Input: part model. Units: mm. Frame: model coordinates. Round coordinates to 2 decimals unless told otherwise and drop trailing zeros. Loops run counter-clockwise (first coordinate to the right, second up) from the corner with the lowest first, then second, coordinate; pieces in that order, holes last. Notation, with made-up numbers: (-32, -29) -> (-15, -29) arc R21 ccw to (-15, 2) -> close; hole circle Ø11 at (-27, -30.75). An arc over 180 degrees is marked (long way). Answer in a Markdown table with one row per item. Add a question column.
Q1. Section A-A, the plane x = -123. Output: boundary loops of the cut face in (y, z) (3 decimals).
Q2. Section C-C, the plane x = 107.5. Output: boundary loops of the cut face in (y, z) (3 decimals).
Q3. Ray query, L1, parallel to Z at x = 114.3, y = 9.5; L2, parallel to X at y = 9.75, z = -78. Return the intervals inside material, ascending. Write a range as from..to.
Q4. Section B-B, the plane y = 10.5. Give the number of separate pieces and of enclosed holes in the cut face, and give its area (3 significant figures).
Q5. Mould query, pull axis X, two halves, no side actions, for faces 1 (the face through (103.77, 7.83, -96.84)), 2 (the face through (-152.4, 8, 8)), 3 (the face through (-2, 0, 5)), 4 (the face through (152.4, 8, 8)). Classes: pulls with the +X half, pulls with the -X half, needs draft (parallel to the pull), parting line crosses it, or undercut.
```python
from build123d import *

# Parameters (mm, degrees)
SKETCH1_W           = 304.8
SKETCH1_H           = 266.7
SKETCH1_R           = 14.2875
BOSS_EXTRUDE1_DEPTH = 15.875
SKETCH2_W           = 304.8
SKETCH2_H           = 12.7
CUT_EXTRUDE1_DEPTH  = 16.875


with BuildPart() as part:
    # Sketch1 → Boss-Extrude1 (new body)
    with BuildSketch(Plane(origin=(0, 0, 0), x_dir=(1, 0, 0), z_dir=(0, 1, 0))):
        Rectangle(SKETCH1_W, SKETCH1_H)
        with Locations((-114.3, 87.180661253)):
            Circle(SKETCH1_R, mode=Mode.SUBTRACT)
        with Locations((114.3, 87.180661253)):
            Circle(SKETCH1_R, mode=Mode.SUBTRACT)
    extrude(amount=BOSS_EXTRUDE1_DEPTH)

    # Sketch2 → Cut-Extrude1 (cut, through all)
    with BuildSketch(Plane(origin=(0, 15.875, 0), x_dir=(1, 0, 0), z_dir=(0, 1, 0))):
        with Locations((0, 127)):
            Rectangle(SKETCH2_W, SKETCH2_H)
    extrude(amount=-CUT_EXTRUDE1_DEPTH, mode=Mode.SUBTRACT)


solid = part.part
```
Answer block:
| question | item | result |
|---|---|---|
| 1 | outline | (0, -120.65) -> (15.875, -120.65) -> (15.875, -98.514) -> (0, -98.514) -> close; (0, -75.847) -> (15.875, -75.847) -> (15.875, 133.35) -> (0, 133.35) -> close |
| 2 | outline | (0, -120.65) -> (15.875, -120.65) -> (15.875, -99.746) -> (0, -99.746) -> close; (0, -74.615) -> (15.875, -74.615) -> (15.875, 133.35) -> (0, 133.35) -> close |
| 3 | L1 | -120.65..-101.47, -72.89..133.35 |
| 3 | L2 | -152.4..-125.25, -103.35..103.35, 125.25..152.4 |
| 4 | separate pieces | 1 |
| 4 | enclosed holes | 2 |
| 4 | area | 76,100 mm^2 |
| 5 | face 1 | undercut |
| 5 | face 2 | pulls with the -X half |
| 5 | face 3 | needs draft |
| 5 | face 4 | pulls with the +X half |
